Verification items for this drawing (mm, ordinates from the low corner). Coordinates: 2 decimals unless noted, no trailing zeros. Order: outer loops, then holes, each group sorted by start corner. A loop starts at its lowest first (then second) coordinate and runs counter-clockwise, first axis right, second up. Notation, with made-up numbers: M 88,-2 L 142,-2 A24 cw 142,36 Z; hole C 49,75 d7. An arc over 180 degrees is marked long. One line per item, written item: value. Start each with the question number.
1) Go/stop test with a flat-tipped pin: P1, Ø6, axis at x = 183.5, z = 19, coming from the +Y side. Record where the tip stops, or that it passes through.
2) Thickness scan on L1, parallel to Z at x = 57, y = 10; L2, parallel to Z at x = 123, y = 120; L3, parallel to X at y = 10, z = 22 (1 decimal). Record the ranges inside material, lowest first. Write a range as from..to.
3) Sectioned sample at A-A, the plane x = 137.5. Enter the section's corners in (y, z), then the cut area to 3 significant figures.
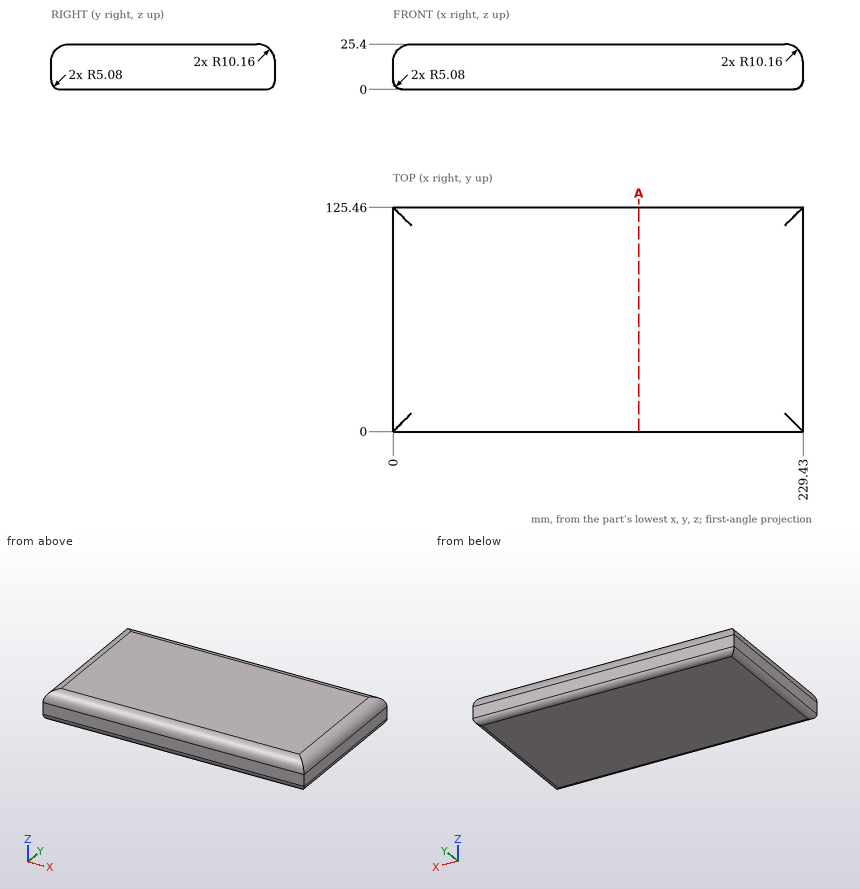
Final values:
1. P1: stops at y = 125.43
2. L1: z = 0..25.4
2. L2: z = 0..24.25
2. L3: x = 2.6..226.9
3. outline: M 0,5.08 A5.08 ccw 5.08,0 L 120.38,0 A5.08 ccw 125.46,5.08 L 125.46,15.24 A10.16 ccw 115.3,25.4 L 10.16,25.4 A10.16 ccw 0,15.24 Z
3. area: 3,130 mm^2
